```python
from build123d import *

# Parameters (mm, degrees)
SKETCH1_W           = 23.898976307
SKETCH1_H           = 24.263846175
BOSS_EXTRUDE3_DEPTH = 13.462
SKETCH2_R           = 7.962435276
CUT_EXTRUDE1_DEPTH  = 35.56
SKETCH3_W           = 22.145451027
SKETCH3_H           = 12.591550695
CUT_EXTRUDE2_DEPTH  = 167.64


with BuildPart() as part:
    # Sketch1 → Boss-Extrude3 (new body)
    with BuildSketch(Plane.XY):
        with Locations((-11.949488154, 12.131923088)):
            Rectangle(SKETCH1_W, SKETCH1_H)
    extrude(amount=BOSS_EXTRUDE3_DEPTH)

    # Sketch2 → Cut-Extrude1 (cut)
    with BuildSketch(Plane.XY.offset(13.462)):
        with Locations((-12.046046864, 8.430505839)):
            Circle(SKETCH2_R)
    extrude(amount=-CUT_EXTRUDE1_DEPTH, mode=Mode.SUBTRACT)

    # Sketch3 → Cut-Extrude2 (cut)
    with BuildSketch(Plane(origin=(0, 24.263846175, 0), x_dir=(1, 0, 0), z_dir=(0, 1, 0))):
        with Locations((-11.63102481, -6.83187996)):
            Rectangle(SKETCH3_W, SKETCH3_H)
    extrude(amount=-CUT_EXTRUDE2_DEPTH, mode=Mode.SUBTRACT)


solid = part.part
```
Geometry check sheet. Reference: the model listing, model coordinates, mm. A direction names the side the tool comes from. Coordinates: 2 decimals unless noted, no trailing zeros. Order: outer loops, then holes, each group sorted by start corner. A loop starts at its lowest first (then second) coordinate and runs counter-clockwise, first axis right, second up. Notation, with made-up numbers: (30.25, -30.5) - (64.25, -30.5) arc R32 cw to (64.25, 2.5) - close; hole circle Ø8 at (42.25, 65.25). An arc over 180 degrees is marked (long way). Use one line per item in the form item = value.
1. Gauge pin test, flat end, axial feed: pin 1 (1 mm diameter, centred on x = -15.5, z = 3, fed in from +Y). Record the tip position at first contact, or that the pin passes through.
Here are the results:
pin_1 = through
2. Section check D-D (y = 5.25). Record the boundary of the cut face in (x, z).
Here are the results:
outline = (-23.9, 0) - (-19.35, 0) - (-19.35, 0.54) - (-22.7, 0.54) - (-22.7, 13.13) - (-19.35, 13.13) - (-19.35, 13.46) - (-23.9, 13.46) - close; (-4.75, 0) - (0, 0) - (0, 13.46) - (-4.75, 13.46) - (-4.75, 13.13) - (-0.56, 13.13) - (-0.56, 0.54) - (-4.75, 0.54) - close
3. Access from +Z, -Z, +X, -X, +Y, -Y to the whole of each face (thin tool, end or side, straight path). Record for faces 1 (the face through (-12, 18, 13.128)), 2 (the face through (-12, 18, 0)).
Here are the results:
face_1 = +Y, -Y
face_2 = -Z, +X, -X, +Y, -Y
4. Section check A-A (z = 10). Record the boundary of the cut face in (x, y), then the cut area to 3 significant figures.
Here are the results:
outline = (-23.9, 0) - (-22.7, 0) - (-22.7, 24.26) - (-23.9, 24.26) - close; (-0.56, 0) - (0, 0) - (0, 24.26) - (-0.56, 24.26) - close
area = 42.5 mm²
5. Section check B-B (x = -3.5). Record the boundary of the cut face in (y, z).
Here are the results:
outline = (0, 0) - (24.26, 0) - (24.26, 0.54) - (0, 0.54) - close; (0, 13.13) - (24.26, 13.13) - (24.26, 13.46) - (0, 13.46) - close
6. Section check C-C (y = 20.25). Record the boundary of the cut face in (x, z).
Here are the results:
outline = (-23.9, 0) - (0, 0) - (0, 13.46) - (-23.9, 13.46) - close; hole (-22.7, 0.54) - (-0.56, 0.54) - (-0.56, 13.13) - (-22.7, 13.13) - close
7. Scan lines: line 1 (Z direction, x = -2.5, y = 8.75); line 2 (X direction, y = 7.5, z = 10.5); line 3 (Y direction, x = -14, z = 0.5). Record each from-to range of solid material in increasing order.
Here are the results:
line_1 = 0 to 0.54, 13.13 to 13.46
line_2 = -23.9 to -22.7, -0.56 to 0
line_3 = 0 to 0.71, 16.15 to 24.26
8. Draft check along Y on faces 3 (the face through (-12, 18, 0.536)), 4 (the face through (-17.915, 13.812, 0.272)), 5 (the face through (-12, 24.264, 0.2)), 6 (the face through (-17.915, 13.812, 13.297)). Enter one of: pulls with the +Y half, pulls with the -Y half, needs draft (parallel to the pull), parting line crosses it, or undercut.
Here are the results:
face_3 = needs draft
face_4 = undercut
face_5 = pulls with the +Y half
face_6 = undercut
